Read the model definition and answer for the solid it produces. Units are mm, in the model's axes. Face numbers are marked on the shaded views. A direction names the side the tool comes from. Coordinates: 2 decimals unless noted, no trailing zeros. Write each loop counter-clockwise with the first axis right and the second up, starting at its lowest first coordinate (ties: lowest second). Pieces come first, ordered by that corner, then holes.
1) The part is cut by section C-C (x = -38). Determine the outline of the cut face in (y, z).
2) The part is cut by section D-D (x = -21). Determine the outline of the cut face in (y, z), then the cut area to 3 significant figures.
3) Which of the six approach directions +Z, -Z, +X, -X, +Y, -Y give full straight-line access (tool end or side, diameter ignored) to the marked faces 1, 2 and 3?
4) Each of these flat-tipped pins is pushed along its axis until it touches: pin 1 Ø13 at (x, z) = (-33.5, 30) entering from +Y; pin 2 Ø1 at (y, z) = (9, 45.5) entering from -X; pin 3 Ø10 at (x, z) = (-35.5, 31) entering from -Y; pin 4 Ø2.5 at (x, z) = (-45.11, 23.44) entering from +Y. Where does it stop, or does it pass through?
5) The part is cut by section B-B (z = 29.5). Determine the outline of the cut face in (x, y).
6) Find the intervals of material crossed by line 1 (X direction, y = 3.25, z = 34.5); line 2 (X direction, y = 10.5, z = 23.5); line 3 (Y direction, x = -29, z = 36), in increasing order.
7) The part is cut by section A-A (y = 16.25). Determine the outline of the cut face in (x, z).
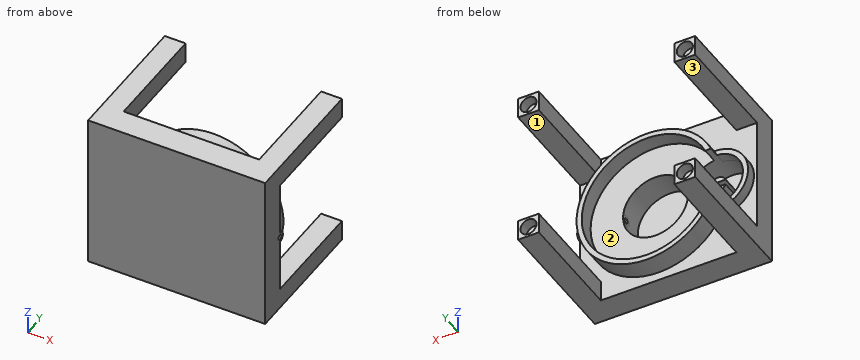
from build123d import *
from build123d.topology import SkipClean

# Parameters (mm, degrees)
SKETCH1_W               = 34.1
SKETCH1_H               = 30.2
BOSS_EXTRUDE1_DEPTH     = 5
SKETCH2_R               = 13.5
BOSS_EXTRUDE2_DEPTH     = 1
SKETCH3_R               = 13.5
SKETCH3_R_2             = 12.5
BOSS_EXTRUDE3_DEPTH     = 3
SKETCH4_R               = 6.25
CUT_EXTRUDE2_DEPTH      = 5
CUT_EXTRUDE3_DEPTH      = 5
CUT_EXTRUDE3_DEPTH_BACK = 5
SKETCH6_R               = 5.4
BOSS_EXTRUDE4_DEPTH     = 2
BOSS_EXTRUDE5_DEPTH     = 4.9
SKETCH10_R              = 1
SKETCH10_R_2            = 0.5
CUT_SWEEP1_START        = -34.728938274
CUT_SWEEP1_OUTLINE_R    = 0.5
CUT_SWEEP1_DEPTH        = 21.723198077
CUT_EXTRUDE4_START      = 5
SKETCH13_R              = 6.25
CUT_EXTRUDE4_DEPTH      = 5
SKETCH14_W              = 4
SKETCH14_H              = 4
BOSS_EXTRUDE6_DEPTH     = 21
SKETCH15_R              = 1.55
CUT_EXTRUDE5_DEPTH      = 2.05


# Read off the part's stored shape, not the designer's step: Cut-Sweep1
with BuildPart() as part:
    # Sketch1 → Boss-Extrude1 (new body)
    with BuildSketch(Plane(origin=(0, 0, 0), x_dir=(1, 0, 0), z_dir=(0, 1, 0))):
        with Locations((-30.055740197, -36.544574539)):
            Rectangle(SKETCH1_W, SKETCH1_H)
    extrude(amount=BOSS_EXTRUDE1_DEPTH)

    # Sketch2 → Boss-Extrude2 (add)
    with BuildSketch(Plane(origin=(0, 5, 0), x_dir=(1, 0, 0), z_dir=(0, 1, 0))):
        with Locations(Location((-28.105740197, -36.544574539, 0), (0, 0, 270))):
            Circle(SKETCH2_R)
    extrude(amount=BOSS_EXTRUDE2_DEPTH)

    # Sketch3 → Boss-Extrude3 (add)
    with BuildSketch(Plane(origin=(0, 6, 0), x_dir=(1, 0, 0), z_dir=(0, 1, 0))):
        with Locations(Location((-28.105740197, -36.544574539, 0), (0, 0, 270))):
            Circle(SKETCH3_R)
        with Locations(Location((-28.105740197, -36.544574539, 0), (0, 0, 270))):
            Circle(SKETCH3_R_2, mode=Mode.SUBTRACT)
    extrude(amount=BOSS_EXTRUDE3_DEPTH)

    # Sketch4 → Cut-Extrude2 (cut)
    with BuildSketch(Plane(origin=(0, 6, 0), x_dir=(1, 0, 0), z_dir=(0, 1, 0))):
        with Locations(Location((-28.105740197, -36.544574539, 0), (0, 0, 270))):
            Circle(SKETCH4_R)
    extrude(amount=-CUT_EXTRUDE2_DEPTH, mode=Mode.SUBTRACT)

    # Sketch6 → Cut-Extrude3 (cut, two sides: drawn at the far end of the back side and taken through both)
    with BuildSketch(Plane(origin=(0, 6, 0), x_dir=(1, 0, 0), z_dir=(0, 1, 0)).offset(-CUT_EXTRUDE3_DEPTH_BACK)):
        with Locations(Location((-40.105740197, -36.544574539, 0), (0, 0, 94.021964573))):
            Circle(SKETCH6_R)
    extrude(amount=CUT_EXTRUDE3_DEPTH + CUT_EXTRUDE3_DEPTH_BACK, mode=Mode.SUBTRACT)

    # Sketch7 → Boss-Extrude4 (add)
    with BuildSketch(Plane(origin=(0, 5, 0), x_dir=(1, 0, 0), z_dir=(0, 1, 0))):
        with BuildLine():
            ThreePointArc((-40.484490197, -41.931275611), (-45.505740197, -36.544574539), (-40.484490197, -31.157873467))
            ThreePointArc((-40.484490197, -31.157873467), (-40.249209884, -30.646596585), (-39.99282353, -30.145570724))
            ThreePointArc((-39.99282353, -30.145570724), (-46.505740197, -36.544574539), (-39.99282353, -42.943578354))
            ThreePointArc((-39.99282353, -42.943578354), (-40.249209884, -42.442552493), (-40.484490197, -41.931275611))
        make_face()
    extrude(amount=BOSS_EXTRUDE4_DEPTH)

    # Sketch9 → Boss-Extrude5 (add)
    with BuildSketch(Plane(origin=(0, 1, 0), x_dir=(1, 0, 0), z_dir=(0, 1, 0))):
        with BuildLine():
            Line((-38.691526635, -37.044574539), (-41.519953759, -37.044574539))
            ThreePointArc((-41.519953759, -37.044574539), (-40.105740197, -38.044574539), (-38.691526635, -37.044574539))
        make_face()
        with BuildLine():
            ThreePointArc((-38.691526635, -36.044574539), (-40.105740197, -35.044574539), (-41.519953759, -36.044574539))
            Line((-41.519953759, -36.044574539), (-38.691526635, -36.044574539))
        make_face()
    extrude(amount=BOSS_EXTRUDE5_DEPTH)

    # Sweep1: sweep along a path in Sketch11
    with BuildLine(Plane(origin=(0, 5, 0), x_dir=(1, 0, 0), z_dir=(0, 1, 0))) as sweep1_path:
        Line((-13.005740197, -36.544574539), (-34.705740197, -36.544574539))
    # Sketch10 → Sweep1 (sweep)
    with BuildSketch(Plane(origin=(-13.005740197, 0, 0), x_dir=(0, 0, -1), z_dir=(1, 0, 0))):
        with Locations((-36.544574539, 5)):
            Circle(SKETCH10_R)
        with Locations((-36.544574539, 5)):
            Circle(SKETCH10_R_2, mode=Mode.SUBTRACT)
    sweep(path=sweep1_path.line)

    # Cut-Sweep1 outline → Cut-Sweep1 (cut)
    with SkipClean():  # the faces are left unmerged after this step: merging them gives an invalid solid
        with BuildSketch(Plane.YZ.offset(CUT_SWEEP1_START)):
            with Locations((5, 36.544574539)):
                Circle(CUT_SWEEP1_OUTLINE_R)
        extrude(amount=CUT_SWEEP1_DEPTH, mode=Mode.SUBTRACT)
    add(part.part.scale(1), mode=Mode.REPLACE)  # the faces are merged on a copy

    # Sketch13 → Cut-Extrude4 (cut)
    with BuildSketch(Plane(origin=(0, 1, 0), x_dir=(1, 0, 0), z_dir=(0, 1, 0)).offset(CUT_EXTRUDE4_START)):
        with Locations(Location((-28.105740197, -36.544574539, 0), (0, 0, 270))):
            Circle(SKETCH13_R)
    extrude(amount=-CUT_EXTRUDE4_DEPTH, mode=Mode.SUBTRACT)

    # Sketch14 → Boss-Extrude6 (add)
    with BuildSketch(Plane(origin=(0, 5, 0), x_dir=(1, 0, 0), z_dir=(0, 1, 0))):
        with Locations((-45.105740197, -23.444574539)):
            Rectangle(SKETCH14_W, SKETCH14_H)
        with Locations((-45.105740197, -49.644574539)):
            Rectangle(SKETCH14_W, SKETCH14_H)
        with Locations((-15.005740197, -49.644574539)):
            Rectangle(SKETCH14_W, SKETCH14_H)
        with Locations((-15.005740197, -23.444574539)):
            Rectangle(SKETCH14_W, SKETCH14_H)
    extrude(amount=BOSS_EXTRUDE6_DEPTH)

    # Sketch15 → Cut-Extrude5 (cut)
    with BuildSketch(Plane(origin=(0, 26, 0), x_dir=(1, 0, 0), z_dir=(0, 1, 0))):
        with Locations(Location((-45.105740197, -49.644574539, 0), (0, 0, 270))):
            Circle(SKETCH15_R)
        with Locations(Location((-45.105740197, -23.444574539, 0), (0, 0, 270))):
            Circle(SKETCH15_R)
        with Locations(Location((-15.005740197, -23.444574539, 0), (0, 0, 270))):
            Circle(SKETCH15_R)
        with Locations(Location((-15.005740197, -49.644574539, 0), (0, 0, 270))):
            Circle(SKETCH15_R)
    extrude(amount=-CUT_EXTRUDE5_DEPTH, mode=Mode.SUBTRACT)


solid = part.part
Reported:
1. outline: (0, 21.44) - (5, 21.44) - (5, 27.36) - (9, 27.36) - (9, 28.91) - (6, 28.91) - (6, 31.57) - (1, 31.57) - (1, 41.52) - (6, 41.52) - (6, 44.18) - (9, 44.18) - (9, 45.73) - (5, 45.73) - (5, 51.64) - (0, 51.64) - close
2. outline: (0, 21.44) - (5, 21.44) - (5, 25.07) - (9, 25.07) - (9, 26.26) - (6, 26.26) - (6, 46.83) - (9, 46.83) - (9, 48.02) - (5, 48.02) - (5, 51.64) - (0, 51.64) - close; hole circle Ø1 at (5, 36.54)
2. area: 180 mm2
3. face 1: +X, +Y
3. face 2: +Y
3. face 3: -X, +Y
4. pin 1: stops at y = 9
4. pin 2: stops at x = -38.63
4. pin 3: stops at y = 0
4. pin 4: stops at y = 23.95
5. outline: (-47.11, 0) - (-13.01, 0) - (-13.01, 5) - (-16.59, 5) - (-16.59, 9) - (-17.78, 9) - (-17.78, 6) - (-38.43, 6) - (-38.43, 9) - (-39.62, 9) - (-39.62, 5) - (-47.11, 5) - close
6. line 1: x = -47.11 to -45.1, -35.11 to -34.01, -22.2 to -13.01
6. line 2: x = -47.11 to -43.11, -17.01 to -13.01
6. line 3: y = 0 to 1
7. outline: (-47.11, 21.44) - (-43.11, 21.44) - (-43.11, 25.44) - (-47.11, 25.44) - close; (-47.11, 47.64) - (-43.11, 47.64) - (-43.11, 51.64) - (-47.11, 51.64) - close; (-17.01, 21.44) - (-13.01, 21.44) - (-13.01, 25.44) - (-17.01, 25.44) - close; (-17.01, 47.64) - (-13.01, 47.64) - (-13.01, 51.64) - (-17.01, 51.64) - close
